from build123d import *

# Parameters (mm, degrees)
SKETCH1_W           = 71
SKETCH1_H           = 200
BOSS_EXTRUDE1_DEPTH = 5
SKETCH2_W           = 65
SKETCH2_H           = 45
BOSS_EXTRUDE3_DEPTH = 2
LPATTERN1_COUNT     = 4
LPATTERN1_PITCH     = 50
SKETCH3_W           = 69
SKETCH3_H           = 49.5
BOSS_EXTRUDE8_DEPTH = 25
LPATTERN5_COUNT     = 4
LPATTERN5_PITCH     = 50


with BuildPart() as part:
    # Sketch1 → Boss-Extrude1 (new body)
    with BuildSketch(Plane(origin=(0, 0, 0), x_dir=(1, 0, 0), z_dir=(0, 1, 0))):
        Rectangle(SKETCH1_W, SKETCH1_H)
    extrude(amount=BOSS_EXTRUDE1_DEPTH)

    # Sketch2 → Boss-Extrude3 (add)
    with BuildSketch(Plane(origin=(0, 5, 0), x_dir=(1, 0, 0), z_dir=(0, 1, 0))):
        with Locations((0, -75)):
            Rectangle(SKETCH2_W, SKETCH2_H)
    boss_extrude3 = extrude(amount=BOSS_EXTRUDE3_DEPTH)

    # LPattern1: Boss-Extrude3 ×4
    with Locations(*[(0, 0, -i * LPATTERN1_PITCH) for i in range(1, LPATTERN1_COUNT)]):
        add(boss_extrude3)

    # Sketch3 → Boss-Extrude8 (add)
    with BuildSketch(Plane(origin=(0, 7, 0), x_dir=(1, 0, 0), z_dir=(0, 1, 0))):
        with Locations((0, -75.25)):
            Rectangle(SKETCH3_W, SKETCH3_H)
    boss_extrude8 = extrude(amount=BOSS_EXTRUDE8_DEPTH)

    # LPattern5: Boss-Extrude8 ×4
    with Locations(*[(0, 0, -i * LPATTERN5_PITCH) for i in range(1, LPATTERN5_COUNT)]):
        add(boss_extrude8)


solid = part.part
Read the model definition and answer for the solid it produces. Units are mm, in the model's axes. A direction names the side the tool comes from. Give positions to 0.01 mm unless a question says otherwise; leave off trailing zeros. Write each loop counter-clockwise with the first axis right and the second up, starting at its lowest first coordinate (ties: lowest second). Pieces come first, ordered by that corner, then holes. Notation, with made-up numbers: (59, 3.25) - (115, 3.25) arc R27 cw to (115, 39.25) - close; hole circle Ø9 at (-2, 8.25). An arc over 180 degrees is marked (long way). Answer in a Markdown table with one row per item. Add a question column.
Item 1: Section A-A, the plane y = 26 is taken. Write down the section's boundary in (x, z).
Item 2: A tool of negligible diameter and unlimited length cuts with its end or side. For faces 1 (the face through (34.5, 19, 26)), 2 (the face through (-34.5, 19, -74)), 3 (the face through (0, 19, -50)), 4 (the face through (-3, 7, -1)), from which of +Z, -Z, +X, -X, +Y, -Y can it reach the whole face along a straight path? Write none if from no direction.
Item 3: Determine the mould class of faces 5 (the face through (0, 2, 100)), 6 (the face through (35.5, 2, 1)), 7 (the face through (-3, 7, 49)) for opening direction Z: pulls with the +Z half, pulls with the -Z half, needs draft (parallel to the pull), parting line crosses it, or undercut.
Item 4: Section B-B, the plane z = -42.5 is taken. Write down the section's boundary in (x, y).
Item 5: Find the intervals of material crossed by L1, parallel to Z at x = -14, y = 9; L2, parallel to X at y = 25.5, z = -18; L3, parallel to X at y = 6, z = 31, in increasing order.
Item 6: Flat-ended cylindrical pins translate along their axes: P1, Ø0.6, axis at y = 6.5, z = -31, coming from the -X side; P2, Ø12.5, axis at x = 16.5, y = 21.5, coming from the -Z side; P3, Ø7.5, axis at y = 16, z = 23, coming from the -X side. Find the tip coordinate at first contact, or state that the pin passes through.
Recorded:
| question | item | result |
|---|---|---|
| 1 | outline | (-34.5, -99.5) - (34.5, -99.5) - (34.5, -50) - (-34.5, -50) - close; (-34.5, -49.5) - (34.5, -49.5) - (34.5, 0) - (-34.5, 0) - close; (-34.5, 0.5) - (34.5, 0.5) - (34.5, 50) - (-34.5, 50) - close; (-34.5, 50.5) - (34.5, 50.5) - (34.5, 100) - (-34.5, 100) - close |
| 2 | face 1 | +Z, -Z, +X, +Y |
| 2 | face 2 | +Z, -Z, -X, +Y |
| 2 | face 3 | +X, -X, +Y |
| 2 | face 4 | none |
| 3 | face 5 | pulls with the +Z half |
| 3 | face 6 | needs draft |
| 3 | face 7 | undercut |
| 4 | outline | (-35.5, 0) - (35.5, 0) - (35.5, 5) - (32.5, 5) - (32.5, 7) - (34.5, 7) - (34.5, 32) - (-34.5, 32) - (-34.5, 7) - (-32.5, 7) - (-32.5, 5) - (-35.5, 5) - close |
| 5 | L1 | z = -99.5 to -50, -49.5 to 0, 0.5 to 50, 50.5 to 100 |
| 5 | L2 | x = -34.5 to 34.5 |
| 5 | L3 | x = -32.5 to 32.5 |
| 6 | P1 | stops at x = -32.5 |
| 6 | P2 | stops at z = -99.5 |
| 6 | P3 | stops at x = -34.5 |
